Verification items for this drawing (mm, ordinates from the low corner). Coordinates: 2 decimals unless noted, no trailing zeros. Order: outer loops, then holes, each group sorted by start corner. A loop starts at its lowest first (then second) coordinate and runs counter-clockwise, first axis right, second up. Notation, with made-up numbers: (21.25, 24.5) -> (50.25, 24.5) arc R27 cw to (50.25, 44.5) -> close; hole circle Ø6 at (-13, 51.5). An arc over 180 degrees is marked (long way). Write each question's results on one line, items separated by ' | '. Start each with the question number.
(1) Draft check along Y on the marked faces 1, 2, 3 and 4. Enter one of: +Y half, -Y half, draft (parallel to the pull), parting line (faces both ways), or undercut.
(2) Cross-section at D-D on x = 40.5. Enter the section's corners in (y, z), and give its area (3 significant figures).
(3) Cross-section at B-B on y = 43.5. Enter the section's corners in (x, z), and give its area (3 significant figures).
(4) Go/stop test with a flat-tipped pin: pin 1 (16 mm diameter, centred on x = 9.5, y = 9.5, fed in from -Z). Record where the tip stops, or that it passes through.
(5) Cross-section at C-C on z = 5.5. Give the number of separate pieces and of enclosed holes in the cut face, and give its area (3 significant figures).
(6) Cross-section at A-A on x = 25. Enter the section's corners in (y, z), and give its area (3 significant figures).
(7) Thickness scan on probe 1 along Y at (x, z) = (40.5, 2.25); probe 2 along X at (y, z) = (36, 1.5); probe 3 along Y at (x, z) = (6.5, 5). Record the ranges inside material, lowest first. Write a range as [from, to].
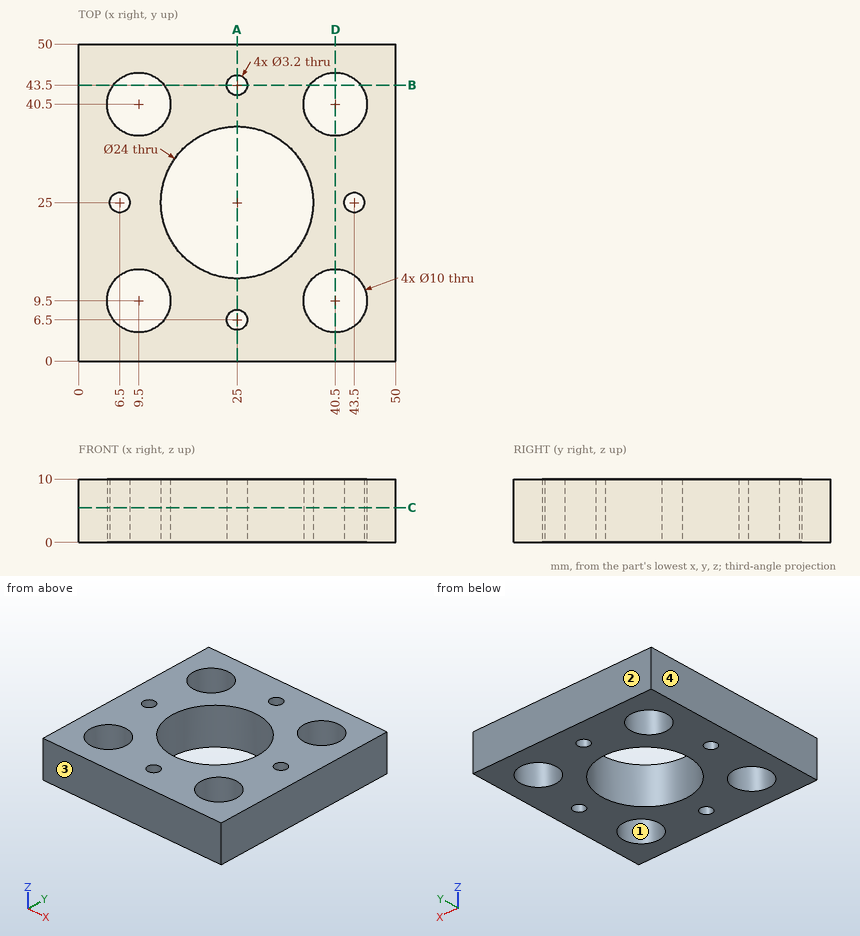
Results are:
1) face 1: undercut | face 2: +Y half | face 3: -Y half | face 4: draft
2) outline: (0, 0) -> (4.5, 0) -> (4.5, 10) -> (0, 10) -> close; (14.5, 0) -> (35.5, 0) -> (35.5, 10) -> (14.5, 10) -> close; (45.5, 0) -> (50, 0) -> (50, 10) -> (45.5, 10) -> close | area: 300 mm2
3) outline: (0, 0) -> (5.5, 0) -> (5.5, 10) -> (0, 10) -> close; (13.5, 0) -> (23.4, 0) -> (23.4, 10) -> (13.5, 10) -> close; (26.6, 0) -> (36.5, 0) -> (36.5, 10) -> (26.6, 10) -> close; (44.5, 0) -> (50, 0) -> (50, 10) -> (44.5, 10) -> close | area: 308 mm2
4) pin 1: stops at z = 0
5) separate pieces: 1 | enclosed holes: 9 | area: 1,700 mm2
6) outline: (0, 0) -> (4.9, 0) -> (4.9, 10) -> (0, 10) -> close; (8.1, 0) -> (13, 0) -> (13, 10) -> (8.1, 10) -> close; (37, 0) -> (41.9, 0) -> (41.9, 10) -> (37, 10) -> close; (45.1, 0) -> (50, 0) -> (50, 10) -> (45.1, 10) -> close | area: 196 mm2
7) probe 1: y = [0, 4.5], [14.5, 35.5], [45.5, 50] | probe 2: x = [0, 7.32], [11.68, 20.2], [29.8, 38.32], [42.68, 50] | probe 3: y = [0, 5.5], [13.5, 23.4], [26.6, 36.5], [44.5, 50]
